Design review of the part built by this model. Coordinates are the model's own, in mm. Coordinates: 2 decimals unless noted, no trailing zeros. Write each loop counter-clockwise with the first axis right and the second up, starting at its lowest first coordinate (ties: lowest second). Pieces come first, ordered by that corner, then holes.
Q1. For probe 1 along Y at (x, z) = (200, 1.1); probe 2 along Y at (x, z) = (199.5, 2.75); probe 3 along Y at (x, z) = (103, 3.85), list the stretches that pass through material, from the lowest coordinate up.
Q2. Take a section at D-D (y = -50). Give the boundary of the cut face in (x, z).
Q3. Take a section at B-B (z = 3.8). Give the boundary of the cut face in (x, y).
Q4. Take a section at C-C (y = 0). Give the boundary of the cut face in (x, z), and give its area (3 significant figures).
Q5. Take a section at A-A (x = 105). Give the boundary of the cut face in (y, z).
Q6. Insertion check: pin 1 (3.5 mm diameter, centred on x = 200, y = 50, fed in from +Z). The pin has a flat end and moves straight along its axis. Give the tip position at first contact, or say it passes through.
```python
from build123d import *

# Parameters (mm, degrees)
EXTRUDE_1_DEPTH     = 5
SKETCH_2_R          = 20
CUT_EXTRUDE_1_DEPTH = 219.46052275
OTHER_1_OUTLINE_R   = 3
OTHER_1_DEPTH       = 5


# Read off the part's stored shape, not the designer's step: 孔1
with BuildPart() as part:
    # 草图1 → 凸台-拉伸1 (new body)
    with BuildSketch(Plane.XY):
        with BuildLine():
            Line((15, 60), (195, 60))
            ThreePointArc((195, 60), (205.606601718, 55.606601718), (210, 45))
            Line((210, 45), (210, -45))
            ThreePointArc((210, -45), (205.606601718, -55.606601718), (195, -60))
            Line((195, -60), (15, -60))
            ThreePointArc((15, -60), (4.393398282, -55.606601718), (0, -45))
            Line((0, -45), (0, 45))
            ThreePointArc((0, 45), (4.393398282, 55.606601718), (15, 60))
        make_face()
    extrude(amount=EXTRUDE_1_DEPTH)

    # 草图2 → 切除-拉伸1 (cut, through all)
    with BuildSketch(Plane.XY.offset(5)):
        with Locations((105, 0)):
            Circle(SKETCH_2_R)
    extrude(amount=-CUT_EXTRUDE_1_DEPTH, mode=Mode.SUBTRACT)

    # 孔1 outline → 孔1 (cut)
    with BuildSketch(Plane.XY):
        with Locations((10, 50)):
            Circle(OTHER_1_OUTLINE_R)
        with Locations((10, -50)):
            Circle(OTHER_1_OUTLINE_R)
        with Locations((200, -50)):
            Circle(OTHER_1_OUTLINE_R)
        with Locations((200, 50)):
            Circle(OTHER_1_OUTLINE_R)
    extrude(amount=OTHER_1_DEPTH, mode=Mode.SUBTRACT)


solid = part.part
```
Response:
1. probe 1: y = -59.14 to -53, -47 to 47, 53 to 59.14
1. probe 2: y = -59.31 to -52.96, -47.04 to 47.04, 52.96 to 59.31
1. probe 3: y = -60 to -19.9, 19.9 to 60
2. outline: (0.86, 0) - (7, 0) - (7, 5) - (0.86, 5) - close; (13, 0) - (197, 0) - (197, 5) - (13, 5) - close; (203, 0) - (209.14, 0) - (209.14, 5) - (203, 5) - close
3. outline: (0, -45) arc R15 ccw to (15, -60) - (195, -60) arc R15 ccw to (210, -45) - (210, 45) arc R15 ccw to (195, 60) - (15, 60) arc R15 ccw to (0, 45) - close; hole circle Ø6 at (10, -50); hole circle Ø6 at (10, 50); hole circle Ø40 at (105, 0); hole circle Ø6 at (200, -50); hole circle Ø6 at (200, 50)
4. outline: (0, 0) - (85, 0) - (85, 5) - (0, 5) - close; (125, 0) - (210, 0) - (210, 5) - (125, 5) - close
4. area: 850 mm2
5. outline: (-60, 0) - (-20, 0) - (-20, 5) - (-60, 5) - close; (20, 0) - (60, 0) - (60, 5) - (20, 5) - close
6. pin 1: passes through
